For this review, take the finished solid that the model builds, in its own axes (mm). A direction names the side the tool comes from. Round coordinates to 2 decimals unless told otherwise and drop trailing zeros. Loops run counter-clockwise (first coordinate to the right, second up) from the corner with the lowest first, then second, coordinate; pieces in that order, holes last.
1. Consider section B-B on y = 4.75. State the section outline as (x, z) points.
2. To check wall thickness, follow line 1 along X through (y, z) = (2.25, -14); line 2 along Y through (x, z) = (1.25, 13); line 3 along Z through (x, y) = (-5.25, 10). State the ranges of each line that lie inside material, in increasing order.
3. Draft analysis for pull direction Y (two halves, no side actions). For faces 1 (the flat face through (0, 0, 0)), 2 (the flat face through (0, 6, 10)), 3 (the flat face through (-4, 1, -12)), state which applies: released by +Y, released by -Y, zero draft, split by the parting line, or undercut.
4. Tool access review of faces 4 (the flat face through (9, 11, -20)), 5 (the flat face through (8, 11, -10)), 6 (the flat face through (0, 1, -4)), 7 (the flat face through (4, 4, 10)): name each direction out of +Z, -Z, +X, -X, +Y, -Y from which nothing blocks a thin tool from reaching the whole face with its end or side.
5. Clearance check with flat-ended pins moving along their axes: pin 1 Ø4 at (x, y) = (-0.5, 14.5) entering from -Z; pin 2 Ø1 at (x, y) = (9.5, 11.5) entering from -Z; pin 3 Ø1.6 at (x, y) = (1, 0.5) entering from -Z. State where each tip first meets the part, or that it passes through.
6. Consider section A-A on z = -9.5. State the section outline as (x, y) points, then the cut area to 3 significant figures.
7. Consider section C-C on z = 7.5. State the section outline as (x, y) points.
8. Consider section D-D on y = 16.75. State the section outline as (x, z) points.
from build123d import *

# Parameters (mm, degrees)
SKETCH_1_W          = 20
SKETCH_1_H          = 40
EXTRUDE_1_DEPTH     = 20
SKETCH_2_W          = 16
SKETCH_2_H          = 20
CUT_EXTRUDE_1_DEPTH = 18
SKETCH_3_W          = 8
SKETCH_3_H          = 38.402735184
CUT_EXTRUDE_2_DEPTH = 20
SKETCH_4_R          = 1
EXTRUDE_2_DEPTH     = 6
SKETCH_5_R          = 1
EXTRUDE_3_DEPTH     = 6
SKETCH_6_W          = 8
SKETCH_6_H          = 4
CUT_EXTRUDE_3_DEPTH = 30


with BuildPart() as part:
    # 草图1 → 凸台-拉伸1 (new body)
    with BuildSketch(Plane(origin=(0, 0, 0), x_dir=(1, 0, 0), z_dir=(0, 1, 0))):
        Rectangle(SKETCH_1_W, SKETCH_1_H)
    extrude(amount=EXTRUDE_1_DEPTH)

    # 草图2 → 切除-拉伸1 (cut)
    with BuildSketch(Plane(origin=(0, 20, 0), x_dir=(1, 0, 0), z_dir=(0, 1, 0))):
        with Locations((0, 10)):
            Rectangle(SKETCH_2_W, SKETCH_2_H)
    extrude(amount=-CUT_EXTRUDE_1_DEPTH, mode=Mode.SUBTRACT)

    # 草图3 → 切除-拉伸2 (cut)
    with BuildSketch(Plane.XZ):
        with Locations((0, -23.201367592)):
            Rectangle(SKETCH_3_W, SKETCH_3_H)
    extrude(amount=-CUT_EXTRUDE_2_DEPTH, mode=Mode.SUBTRACT)

    # 草图4 → 凸台-拉伸2 (add)
    with BuildSketch(Plane(origin=(-4, 0, 0), x_dir=(0, 0, -1), z_dir=(1, 0, 0))):
        with Locations((20, 1)):
            Circle(SKETCH_4_R)
    extrude(amount=-EXTRUDE_2_DEPTH)

    # 草图5 → 凸台-拉伸3 (add)
    with BuildSketch(Plane.ZY.offset(-4)):
        with Locations((-20, 1)):
            Circle(SKETCH_5_R)
    extrude(amount=-EXTRUDE_3_DEPTH)

    # 草图6 → 切除-拉伸3 (cut)
    with BuildSketch(Plane(origin=(0, 0, 0), x_dir=(-1, 0, 0), z_dir=(0, 0, -1))):
        with Locations((0, 4)):
            Rectangle(SKETCH_6_W, SKETCH_6_H)
    extrude(amount=-CUT_EXTRUDE_3_DEPTH, mode=Mode.SUBTRACT)


solid = part.part
Resolved:
1. outline: (-10, -20) - (-8, -20) - (-8, 0) - (-4, 0) - (-4, 20) - (-10, 20) - close; (4, 0) - (8, 0) - (8, -20) - (10, -20) - (10, 20) - (4, 20) - close
2. line 1: x = -10 to -8, 8 to 10
2. line 2: y = 0 to 2, 6 to 20
2. line 3: z = 0 to 20
3. face 1: released by -Y
3. face 2: undercut
3. face 3: zero draft
4. face 4: -Z, +X, -X, +Y
4. face 5: -Z, +Y
4. face 6: -Z, +Y, -Y
4. face 7: +Z, -Z
5. pin 1: stops at z = 0
5. pin 2: stops at z = -20
5. pin 3: stops at z = -4
6. outline: (-10, 0) - (-4, 0) - (-4, 2) - (-8, 2) - (-8, 20) - (-10, 20) - close; (4, 0) - (10, 0) - (10, 20) - (8, 20) - (8, 2) - (4, 2) - close
6. area: 96.0 mm2
7. outline: (-10, 0) - (10, 0) - (10, 20) - (-10, 20) - close; hole (-4, 2) - (4, 2) - (4, 6) - (-4, 6) - close
8. outline: (-10, -20) - (-8, -20) - (-8, 0) - (8, 0) - (8, -20) - (10, -20) - (10, 20) - (-10, 20) - close
